Could you check a few things on this model? Use its own coordinates, in mm. Coordinates: 2 decimals unless noted, no trailing zeros. Order: outer loops, then holes, each group sorted by start corner. A loop starts at its lowest first (then second) coordinate and runs counter-clockwise, first axis right, second up. Notation, with made-up numbers: (6.5, 32.5) -> (42.5, 32.5) arc R25 ccw to (42.5, 49.5) -> close; hole circle Ø9 at (40, 7). An arc over 180 degrees is marked (long way). Return JSON: item names as keys, results as strings. Group by question number.
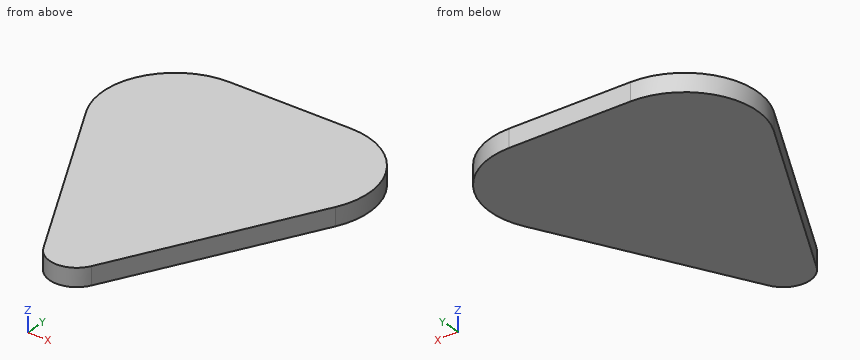
from build123d import *

# Parameters (mm, degrees)
F1_DEPTH = 1


# Not quite as in the source:
# - a feature of the source that left no trace in its solid (it failed there, or was rolled back) is left out


with BuildPart() as f1:
    # F0 (on Top) → F1 (new body, symmetric)
    with BuildSketch(Plane.XY):
        with BuildLine():
            Line((6.7490902932, 12.4546424842), (-6.7490902932, 12.4546424842))
            ThreePointArc((-6.7490902932, 12.4546424842), (-13.5977314614, 8.5893872344), (-13.8284360723, 0.7286710215))
            Line((-13.8284360723, 0.7286710215), (-2.6547546671, -20.5013236482))
            ThreePointArc((-2.6547546671, -20.5013236482), (0, -22.1040843497), (2.6547546671, -20.5013236482))
            Line((2.6547546671, -20.5013236482), (13.8284360723, 0.7286710215))
            ThreePointArc((13.8284360723, 0.7286710215), (13.5977314614, 8.5893872344), (6.7490902932, 12.4546424842))
        make_face()
    extrude(amount=F1_DEPTH, both=True)


solid = f1.part
Q1. I want a section at B-B on y = -9. Please give me the cut outline in (x, z).
Q2. I'm going to push a flat-ended pin straight in: pin 1 Ø2 at (x, y) = (11, -5) entering from -Z. Where does the tip first touch, or does it pass through?
Q3. I want a section at C-C on x = -2. Please give me the cut outline in (y, z), and give its area (3 significant figures).
Q4. I want a section at A-A on z = 0.65. Please give me the cut outline in (x, y), and give its area (3 significant figures).
Q5. I need wall thicknesses on line 1 along X through (y, z) = (4, -0.55); line 2 along Y through (x, z) = (0.25, 0.95); line 3 along X through (y, z) = (-1.5, -0.75). Which ranges of each line are inside material? Lowest first, please. Write a range as from..to.
Response values:
{
 "1": {"outline": "(-8.71, -1) -> (8.71, -1) -> (8.71, 1) -> (-8.71, 1) -> close"},
 "2": {"pin 1": "stops at z = -1"},
 "3": {"outline": "(-21.34, -1) -> (12.45, -1) -> (12.45, 1) -> (-21.34, 1) -> close", "area": "67.6 mm²"},
 "4": {"outline": "(-13.83, 0.73) -> (-2.65, -20.5) arc R3 ccw to (2.65, -20.5) -> (13.83, 0.73) arc R8 ccw to (6.75, 12.45) -> (-6.75, 12.45) arc R8 ccw to start", "area": "672 mm²"},
 "5": {"line 1": "x = -14.74..14.74", "line 2": "y = -22.09..12.45", "line 3": "x = -12.66..12.66"}
}
